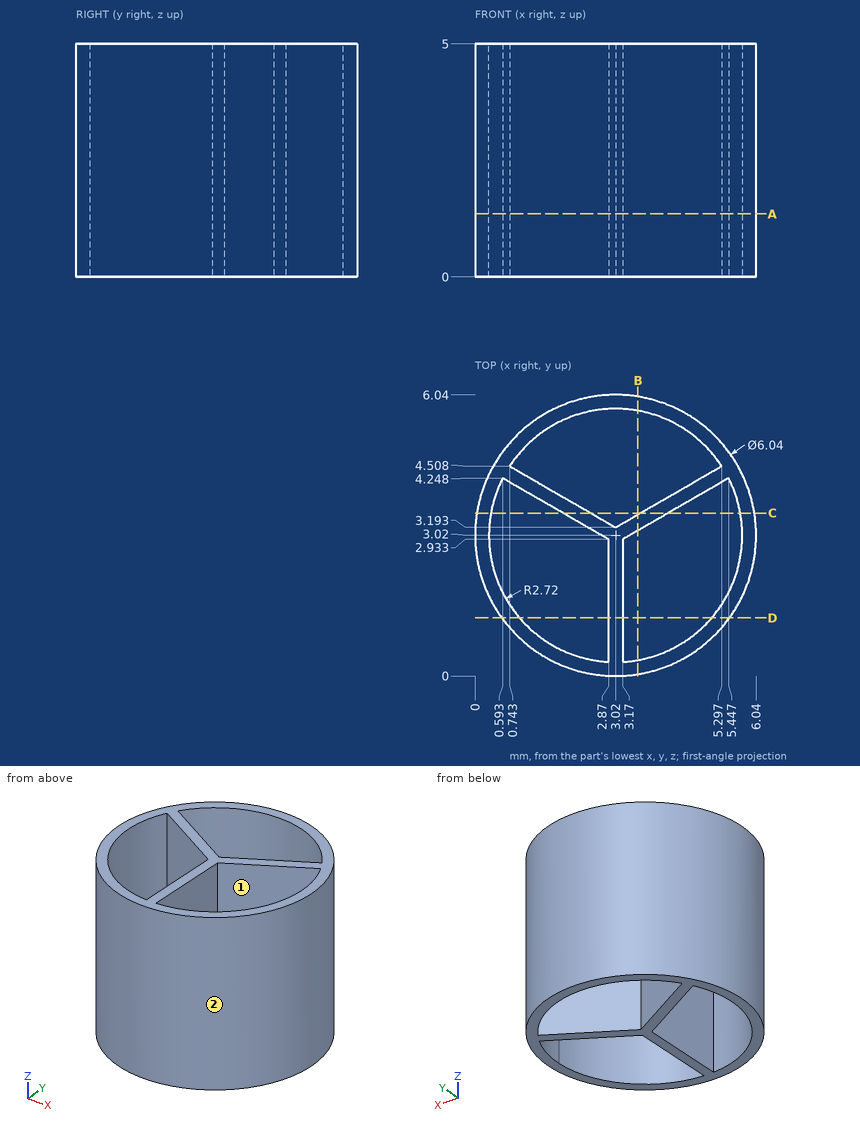
Could you check a few things on this drawing? It's one solid part, dimensions in mm from its lowest x, y, z. Give positions to 0.01 mm unless a question says otherwise; leave off trailing zeros. Write each loop counter-clockwise with the first axis right and the second up, starting at its lowest first coordinate (ties: lowest second). Pieces come first, ordered by that corner, then holes. Notation, with made-up numbers: (9, 45) -> (19, 45) arc R28 ccw to (19, 80) -> close; hole circle Ø9 at (32.5, 47). An arc over 180 degrees is marked (long way). Write item = value, one per line.
(1) Suppose I cut it at D-D on y = 1.25. Count the separate pieces of the cut face and the enclosed holes in it.
Worked out:
separate_pieces = 3
enclosed_holes = 0
(2) Suppose I cut it at A-A on z = 1.35. Write out the boundary of the cut face in (x, y).
Worked out:
outline = circle Ø6.04 at (3.02, 3.02); hole (0.59, 4.25) arc R2.72 ccw to (2.87, 0.3) -> (2.87, 2.93) -> close; hole (0.74, 4.51) -> (3.02, 3.19) -> (5.3, 4.51) arc R2.72 ccw to start; hole (3.17, 0.3) arc R2.72 ccw to (5.45, 4.25) -> (3.17, 2.93) -> close
(3) Thinking about a two-plate mould opening in Y: for the marked faces 1 and 2, which applies, released by +Y, released by -Y, zero draft, split by the parting line, or undercut?
Worked out:
face_1 = undercut
face_2 = split by the parting line
(4) Suppose I cut it at C-C on y = 3.5. Write out the boundary of the cut face in (x, z).
Worked out:
outline = (0.04, 0) -> (0.34, 0) -> (0.34, 5) -> (0.04, 5) -> close; (1.89, 0) -> (2.49, 0) -> (2.49, 5) -> (1.89, 5) -> close; (3.55, 0) -> (4.15, 0) -> (4.15, 5) -> (3.55, 5) -> close; (5.7, 0) -> (6, 0) -> (6, 5) -> (5.7, 5) -> close
(5) Suppose I cut it at B-B on x = 3.5. Write out the boundary of the cut face in (y, z).
Worked out:
outline = (0.04, 0) -> (0.34, 0) -> (0.34, 5) -> (0.04, 5) -> close; (3.12, 0) -> (3.47, 0) -> (3.47, 5) -> (3.12, 5) -> close; (5.7, 0) -> (6, 0) -> (6, 5) -> (5.7, 5) -> close
(6) I need wall thicknesses on probe 1 along X at (y, z) = (1.5, 3.3) (1 decimal); probe 2 along X at (y, z) = (2, 3.3); probe 3 along Y at (x, z) = (3.5, 3.9) (1 decimal). Which ranges of each line are inside material? Lowest first, please. Write a range as from..to.
Worked out:
probe_1 = 0.4..0.8, 2.9..3.2, 5.3..5.6
probe_2 = 0.18..0.5, 2.87..3.17, 5.54..5.86
probe_3 = 0..0.3, 3.1..3.5, 5.7..6
(7) I'm going to push flat-ended pins straight in: P1, Ø3, axis at y = 1, z = 1.5, coming from the +X side (1 decimal); P2, Ø2, axis at y = 1, z = 3.5, coming from the -X side; P3, Ø1, axis at y = 5, z = 1.5, coming from the +X side. Where does each tip first touch, or does it pass through?
Worked out:
P1 = 6
P2 = 0.18
P3 = 5.65
